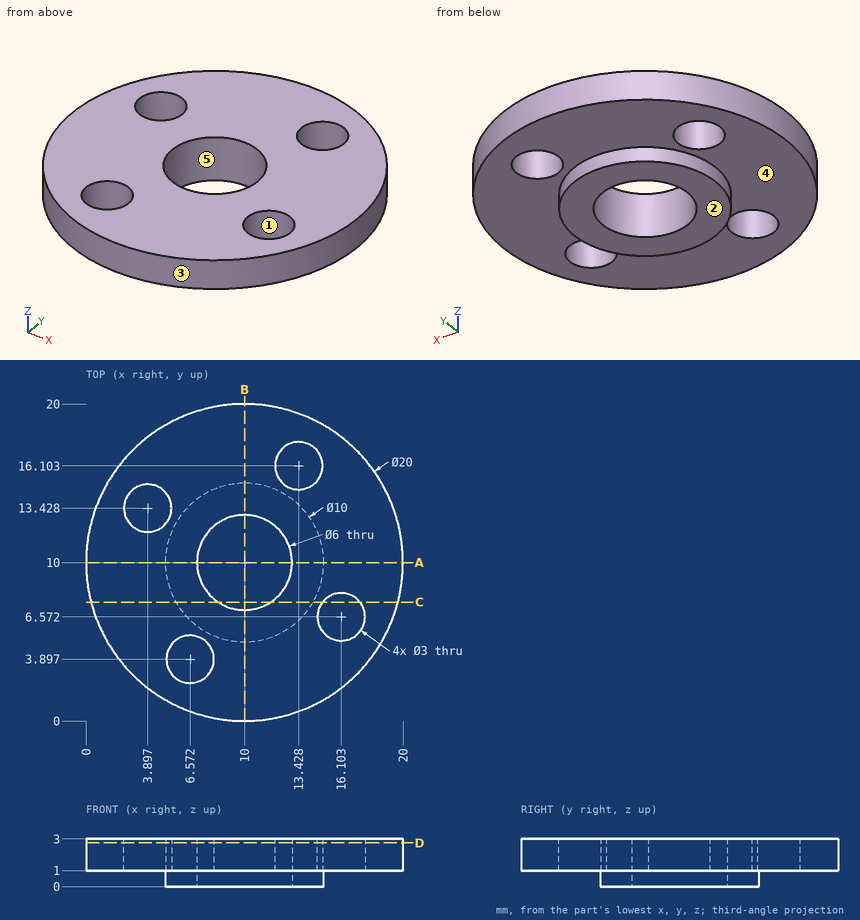
Input: dimensioned drawing with shaded views. Units: mm. Origin: part minimum x, y, z. A direction names the side the tool comes from. Give positions to 0.01 mm unless a question says otherwise; leave off trailing zeros. Order: outer loops, then holes, each group sorted by start corner. A loop starts at its lowest first (then second) coordinate and runs counter-clockwise, first axis right, second up. Notation, with made-up numbers: (-39.5, 55) -> (-35.5, 55) arc R22 ccw to (-35.5, 67) -> close; hole circle Ø2 at (-11, 84). An arc over 180 degrees is marked (long way). Use a Markdown table: item, result.
1) Contact query for flat-ended pins moving along their axis: P1, Ø10, axis at x = 17, y = 13.5, coming from the -Z side; P2, Ø1, axis at y = 8, z = 2, coming from the -X side; P3, Ø5, axis at x = 15, y = 18, coming from the -Z side; P4, Ø1.5, axis at y = 13, z = 2, coming from the -X side. Output: stop coordinate, or through.
Answer list:
| item | result |
|---|---|
| P1 | z = 0 |
| P2 | x = 0.11 |
| P3 | z = 1 |
| P4 | x = 0.26 |
2) Mould query, pull axis X, two halves, no side actions, for the marked faces 1, 2 and 3. Classes: +X half, -X half, draft (parallel to the pull), parting line (faces both ways), or undercut.
Answer list:
| item | result |
|---|---|
| face 1 | undercut |
| face 2 | draft |
| face 3 | parting line |
3) Section query A-A, the plane y = 10. Return the cut outline in (x, z), then the cut area to 3 significant figures.
Answer list:
| item | result |
|---|---|
| outline | (0, 1) -> (5, 1) -> (5, 0) -> (7, 0) -> (7, 3) -> (0, 3) -> close; (13, 0) -> (15, 0) -> (15, 1) -> (20, 1) -> (20, 3) -> (13, 3) -> close |
| area | 32.0 mm² |
4) Ray query, line 1 along Y through (x, z) = (12.5, 1.7) (1 decimal); line 2 along Y through (x, z) = (10, 2.3); line 3 along X through (y, z) = (7.75, 1.55) (1 decimal). Return the intervals inside material, ascending. Write a range as [from, to].
Answer list:
| item | result |
|---|---|
| line 1 | [0.3, 8.3], [11.7, 14.9], [17.3, 19.7] |
| line 2 | [0, 7], [13, 20] |
| line 3 | [0.3, 8], [12, 15.2], [17, 19.7] |
5) Reachability of the marked faces 4 and 5 from +Z, -Z, +X, -X, +Y, -Y: full face, straight path, thin tool, end or side. Return the list, or none.
Answer list:
| item | result |
|---|---|
| face 4 | -Z |
| face 5 | +Z, -Z |
6) Section query C-C, the plane y = 7.5. Return the cut outline in (x, z) (1 decimal).
Answer list:
| item | result |
|---|---|
| outline | (0.3, 1) -> (5.7, 1) -> (5.7, 0) -> (8.3, 0) -> (8.3, 3) -> (0.3, 3) -> close; (11.7, 0) -> (14.3, 0) -> (14.3, 1) -> (14.9, 1) -> (14.9, 3) -> (11.7, 3) -> close; (17.3, 1) -> (19.7, 1) -> (19.7, 3) -> (17.3, 3) -> close |
7) Section query D-D, the plane z = 2.75. Return the cut outline in (x, y), then the cut area to 3 significant figures.
Answer list:
| item | result |
|---|---|
| outline | circle Ø20 at (10, 10); hole circle Ø3 at (3.9, 13.43); hole circle Ø3 at (6.57, 3.9); hole circle Ø6 at (10, 10); hole circle Ø3 at (13.43, 16.1); hole circle Ø3 at (16.1, 6.57) |
| area | 258 mm² |
